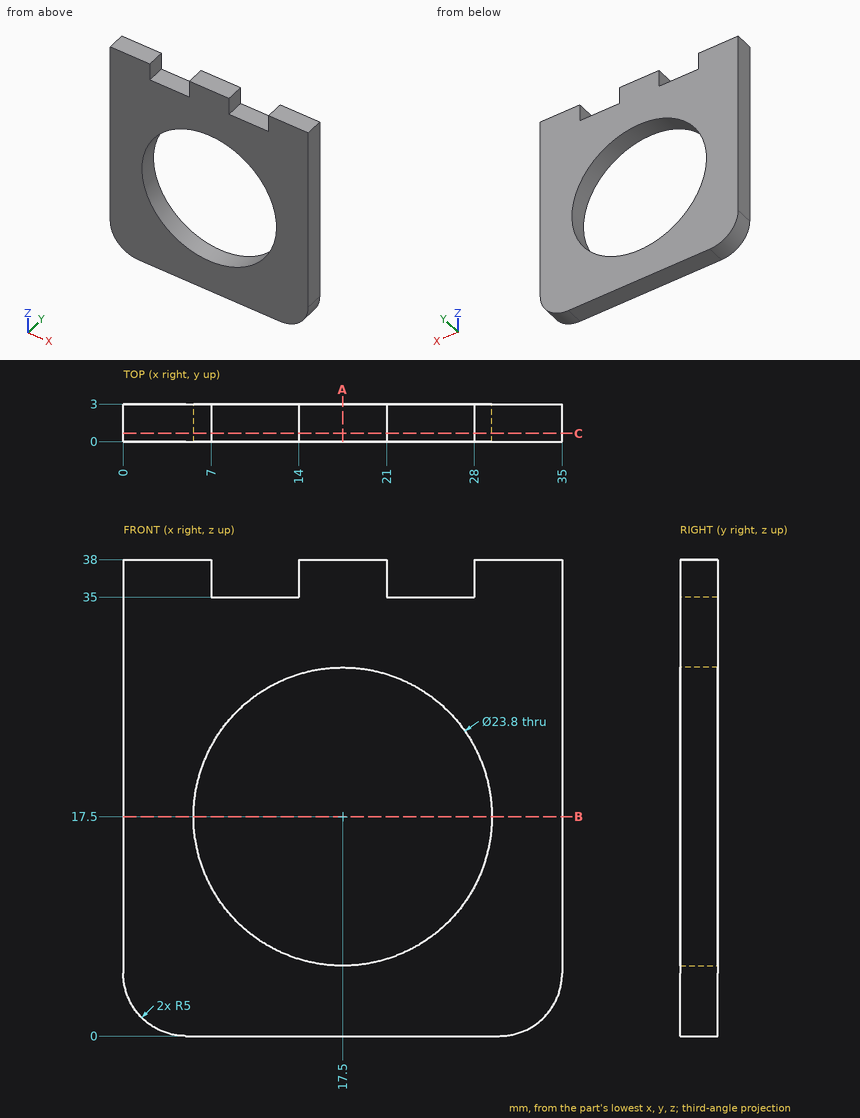
Job drawing, mm, ordinate dimensions from the low corner. One solid piece. Coordinates: 2 decimals unless noted, no trailing zeros. Order: outer loops, then holes, each group sorted by start corner. A loop starts at its lowest first (then second) coordinate and runs counter-clockwise, first axis right, second up. Notation, with made-up numbers: M 73.25,-13.75 L 106.25,-13.75 A17 cw 106.25,-7.75 Z; hole C 3.25,-22.75 d3. An arc over 180 degrees is marked long. Return JSON: item names as keys, results as strings.
1. Saw through at A-A (x = 17.5). Give the cut face in (y, z), and give its area (3 significant figures).
Ans:
{"outline": "M 0,0 L 3,0 L 3,5.6 L 0,5.6 Z; M 0,29.4 L 3,29.4 L 3,38 L 0,38 Z", "area": "42.6 mm^2"}
2. Flat gauge pins, fed straight in: pin 1 (3 mm diameter, centred on x = 9, z = 25, fed in from -Y); pin 2 (19 mm diameter, centred on x = 17.5, z = 17.5, fed in from +Y); pin 3 (1.5 mm diameter, centred on x = 11, y = 1.5, fed in from +Z). Where does each tip first touch, or does it go through?
Ans:
{"pin 1": "y = 0", "pin 2": "through", "pin 3": "z = 35"}
3. Saw through at B-B (z = 17.5). Give the cut face in (x, y), and give its area (3 significant figures).
Ans:
{"outline": "M 0,0 L 5.6,0 L 5.6,3 L 0,3 Z; M 29.4,0 L 35,0 L 35,3 L 29.4,3 Z", "area": "33.6 mm^2"}
4. Saw through at C-C (y = 0.65). Give the cut face in (x, z), and give its area (3 significant figures).
Ans:
{"outline": "M 0,5 A5 ccw 5,0 L 30,0 A5 ccw 35,5 L 35,38 L 28,38 L 28,35 L 21,35 L 21,38 L 14,38 L 14,35 L 7,35 L 7,38 L 0,38 Z; hole C 17.5,17.5 d23.8", "area": "832 mm^2"}
5. Drill centre lines: probe 1 along X at (y, z) = (2, 36.5); probe 2 along X at (y, z) = (2.1, 17.5); probe 3 along Z at (x, y) = (16.5, 2.8). Where is each one in solid material? Low to high.
Ans:
{"probe 1": "0 to 7, 14 to 21, 28 to 35", "probe 2": "0 to 5.6, 29.4 to 35", "probe 3": "0 to 5.64, 29.36 to 38"}
